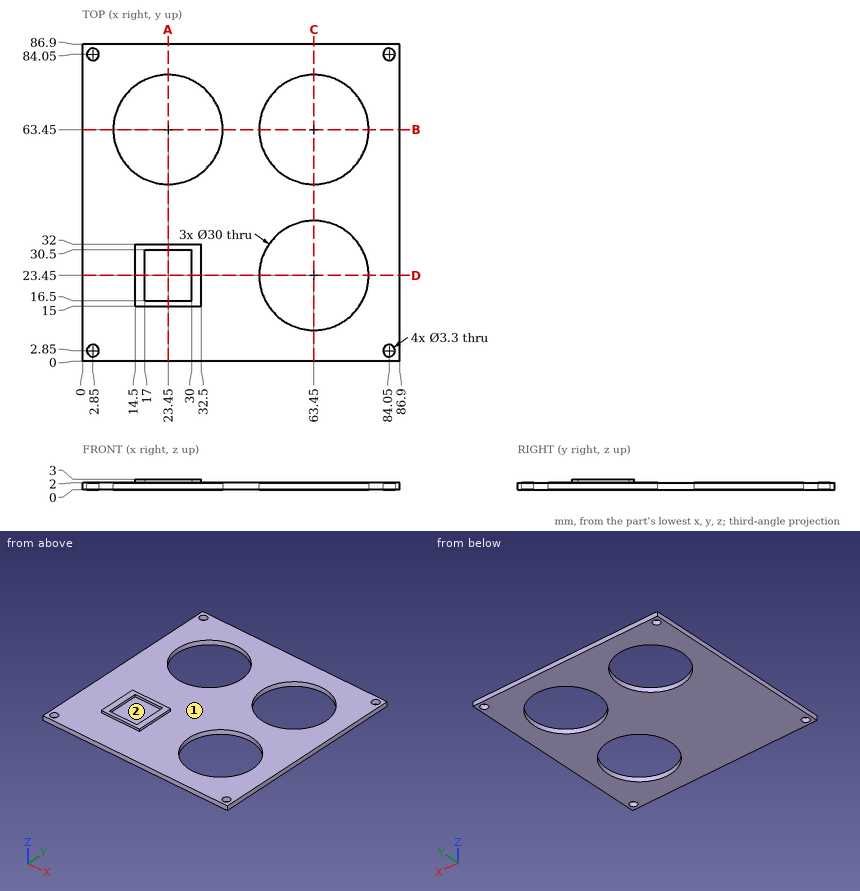
Check sheet for the drawn part. Datum: minimum x, y, z corner. Units: mm. Coordinates: 2 decimals unless noted, no trailing zeros. Loops run counter-clockwise (first coordinate to the right, second up) from the corner with the lowest first, then second, coordinate; pieces in that order, holes last. Notation, with made-up numbers: (62, -15.5) -> (85, -15.5) arc R22 ccw to (85, -0.5) -> close; hole circle Ø10 at (23, 26). An arc over 180 degrees is marked (long way). Answer in a Markdown table with one row per item.
1) Draft check along X on the marked faces 1 and 2. Enter one of: released by +X, released by -X, zero draft, split by the parting line, or undercut.
The answers:
| item | result |
|---|---|
| face 1 | zero draft |
| face 2 | undercut |
2) Section check B-B (y = 63.45). Record the cut outline in (x, z), and give its area (3 significant figures).
The answers:
| item | result |
|---|---|
| outline | (0, 0) -> (8.45, 0) -> (8.45, 2) -> (0, 2) -> close; (38.45, 0) -> (48.45, 0) -> (48.45, 2) -> (38.45, 2) -> close; (78.45, 0) -> (86.9, 0) -> (86.9, 2) -> (78.45, 2) -> close |
| area | 53.8 mm2 |
3) Section check D-D (y = 23.45). Record the cut outline in (x, z).
The answers:
| item | result |
|---|---|
| outline | (0, 0) -> (48.45, 0) -> (48.45, 2) -> (32.5, 2) -> (32.5, 3) -> (30, 3) -> (30, 2) -> (17, 2) -> (17, 3) -> (14.5, 3) -> (14.5, 2) -> (0, 2) -> close; (78.45, 0) -> (86.9, 0) -> (86.9, 2) -> (78.45, 2) -> close |
4) Section check A-A (x = 23.45). Record the cut outline in (y, z).
The answers:
| item | result |
|---|---|
| outline | (0, 0) -> (48.45, 0) -> (48.45, 2) -> (32, 2) -> (32, 3) -> (30.5, 3) -> (30.5, 2) -> (16.5, 2) -> (16.5, 3) -> (15, 3) -> (15, 2) -> (0, 2) -> close; (78.45, 0) -> (86.9, 0) -> (86.9, 2) -> (78.45, 2) -> close |
5) Scan lines: line 1 along X through (y, z) = (84.05, 0.8); line 2 along Y through (x, z) = (63.45, 0.7). Record each from-to range of solid material in increasing order. Write a range as from..to.
The answers:
| item | result |
|---|---|
| line 1 | x = 0..1.2, 4.5..82.4, 85.7..86.9 |
| line 2 | y = 0..8.45, 38.45..48.45, 78.45..86.9 |
6) Depth check by flat-ended pin: P1, Ø3, axis at x = 2.85, y = 84.05, coming from the -Z side; P2, Ø0.5, axis at x = 23.5, z = 2.5, coming from the -Y side; P3, Ø12, axis at x = 21, y = 75.5, coming from the +Z side. Enter the tip coordinate at first touch or a pass-through.
The answers:
| item | result |
|---|---|
| P1 | passes through |
| P2 | stops at y = 15 |
| P3 | stops at z = 2 |
